Model file for the job. Use its own axes, mm. Face numbers are marked on the shaded views. A direction names the side the tool comes from. Round coordinates to 2 decimals unless told otherwise and drop trailing zeros. Loops run counter-clockwise (first coordinate to the right, second up) from the corner with the lowest first, then second, coordinate; pieces in that order, holes last. Notation, with made-up numbers: M 84,-19.75 L 97,-19.75 A13 ccw 97,4.25 Z; hole C 3,16 d5. An arc over 180 degrees is marked long. Use a Markdown table: item, result. Add a question column.
Q1. Mould opens along Y. For the marked faces 1, 2 and 3 say: +Y half, -Y half, draft (parallel to the pull), parting line (faces both ways), or undercut.
Q2. Cut at A-A (z = 17). Give the cut face in (x, y).
Q3. Cut at B-B (y = 10). Give the cut face in (x, z).
Q4. Cut at C-C (x = 131). Give the cut face in (y, z), plus the area to 3 significant figures.
Q5. Probe line 1 (Y direction, x = 25, z = 54); line 2 (X direction, y = 14.5, z = 6); line 3 (Z direction, x = 43, y = 40). List the from-to ranges inside material, lowest first. Write a range as from..to.
Q6. Tool access for the marked faces 4, 5, 6, 7 and 8: list every direction of +Z, -Z, +X, -X, +Y, -Y with a clear straight run to the whole face (end or side of a thin tool).
Q7. Pin check, flat tips, straight feed: pin 1 (6 mm diameter, centred on y = 31.5, z = 79, fed in from +X); pin 2 (20.5 mm diameter, centred on y = 28.5, z = 11.5, fed in from +X); pin 3 (9.5 mm diameter, centred on x = 78.5, y = 25.5, fed in from -Z); pin 4 (12 mm diameter, centred on x = 118.5, y = 7, fed in from -Z). Stop position of each tip, or through.
Q8. Cut at D-D (y = 47.5). Give the cut face in (x, z).
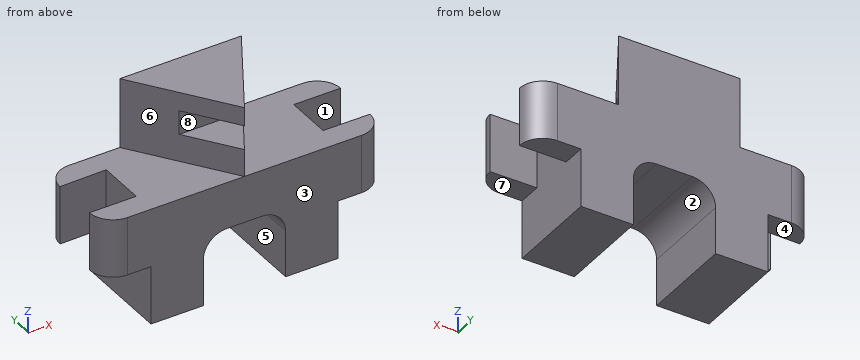
from build123d import *

# Parameters (mm, degrees)
F2_DEPTH = 50.8
F3_DEPTH = 63.5
F5_START = 38.1
F5_DEPTH = 63.5
F6_W     = 26.5905056149
F6_H     = 13.1163969636
F7_DEPTH = 152.401


with BuildPart() as f2:
    # F0 (on Front) → F2 (new body)
    with BuildSketch(Plane.XZ):
        with BuildLine():
            Line((25.4, 31.75), (25.4, 0))
            Line((25.4, 0), (53.848, 0))
            Line((53.848, 0), (53.848, 25.4))
            ThreePointArc((53.848, 25.4), (57.5677438789, 34.3802561211), (66.548, 38.1))
            Line((66.548, 38.1), (85.852, 38.1))
            ThreePointArc((85.852, 38.1), (94.8322561211, 34.3802561211), (98.552, 25.4))
            Line((98.552, 25.4), (98.552, 0))
            Line((98.552, 0), (127, 0))
            Line((127, 0), (127, 31.75))
            Line((127, 31.75), (152.4, 31.75))
            Line((152.4, 31.75), (152.4, 63.5))
            Line((152.4, 63.5), (127, 63.5))
            Line((127, 63.5), (88.9, 63.5))
            Line((88.9, 63.5), (63.5, 63.5))
            Line((63.5, 63.5), (38.1, 63.5))
            Line((38.1, 63.5), (25.4, 63.5))
            Line((25.4, 63.5), (0, 63.5))
            Line((0, 63.5), (0, 31.75))
            Line((0, 31.75), (25.4, 31.75))
        make_face()
    extrude(amount=-F2_DEPTH)

    # F1 (on Top) → F3 (cut)
    with BuildSketch(Plane.XY):
        with BuildLine():
            Line((0, 50.8), (0, 38.1))
            ThreePointArc((0, 38.1), (3.7197438789, 47.0802561211), (12.7, 50.8))
            Line((12.7, 50.8), (0, 50.8))
        make_face()
        with BuildLine():
            ThreePointArc((12.7, 0), (3.7197438789, 3.7197438789), (0, 12.7))
            Line((0, 12.7), (0, 0))
            Line((0, 0), (12.7, 0))
        make_face()
        Polygon((0, 38.1), (0, 12.7), (25.4, 12.7), (25.4, 38.5738648474), align=None)
        Polygon((127, 12.8180403262), (152.4, 12.7), (152.4, 38.1), (127, 38.1), align=None)
        with BuildLine():
            Line((152.4, 0), (152.4, 12.7))
            ThreePointArc((152.4, 12.7), (148.6802561211, 3.7197438789), (139.7, 0))
            Line((139.7, 0), (152.4, 0))
        make_face()
        with BuildLine():
            ThreePointArc((139.7, 50.8), (148.6802561211, 47.0802561211), (152.4, 38.1))
            Line((152.4, 38.1), (152.4, 50.8))
            Line((152.4, 50.8), (139.7, 50.8))
        make_face()
    extrude(amount=F3_DEPTH, mode=Mode.SUBTRACT)

    # F4 (on Top) → F5 (join)
    with BuildSketch(Plane.XY.offset(F5_START)):
        Polygon((40.4607152585, 50.8), (76.2, 0), (106.5007152585, 50.8), align=None)
    extrude(amount=F5_DEPTH)

    # F6 (on Right) → F7 (cut, through all)
    with BuildSketch(Plane.YZ):
        with Locations((13.2952528074, 84.9594064057)):
            Rectangle(F6_W, F6_H)
    extrude(amount=F7_DEPTH, mode=Mode.SUBTRACT)


solid = f2.part
Checked values:
| question | item | result |
|---|---|---|
| 1 | face 1 | undercut |
| 1 | face 2 | draft |
| 1 | face 3 | -Y half |
| 2 | outline | M 25.4,0 L 53.85,0 L 53.85,50.8 L 25.4,50.8 Z; M 98.55,0 L 127,0 L 127,50.8 L 98.55,50.8 Z |
| 3 | outline | M 0.29,31.75 L 25.4,31.75 L 25.4,0 L 53.85,0 L 53.85,25.4 A12.7 cw 66.55,38.1 L 85.85,38.1 A12.7 cw 98.55,25.4 L 98.55,0 L 127,0 L 127,31.75 L 152.11,31.75 L 152.11,63.5 L 82.16,63.5 L 82.16,78.4 L 69.16,78.4 L 69.16,63.5 L 0.29,63.5 Z; M 69.16,91.52 L 82.16,91.52 L 82.16,101.6 L 69.16,101.6 Z |
| 4 | outline | M 0,31.75 L 12.8,31.75 L 12.8,63.5 L 0,63.5 Z; M 38.1,31.75 L 50.8,31.75 L 50.8,63.5 L 38.1,63.5 Z |
| 4 | area | 810 mm^2 |
| 5 | line 1 | y = 0..12.7, 38.57..50.8 |
| 5 | line 2 | x = 25.4..53.85, 98.55..127 |
| 5 | line 3 | z = 0..63.5 |
| 6 | face 4 | -Z, -X, +Y, -Y |
| 6 | face 5 | -Z, +Y, -Y |
| 6 | face 6 | +Z, -X, -Y |
| 6 | face 7 | -Z, +X, +Y, -Y |
| 6 | face 8 | +X, -X, -Y |
| 7 | pin 1 | stops at x = 96.78 |
| 7 | pin 2 | stops at x = 127 |
| 7 | pin 3 | stops at z = 38.1 |
| 7 | pin 4 | stops at z = 0 |
| 8 | outline | M 4.16,31.75 L 25.4,31.75 L 25.4,0 L 53.85,0 L 53.85,25.4 A12.7 cw 66.55,38.1 L 85.85,38.1 A12.7 cw 98.55,25.4 L 98.55,0 L 127,0 L 127,31.75 L 148.24,31.75 L 148.24,63.5 L 104.53,63.5 L 104.53,101.6 L 42.78,101.6 L 42.78,63.5 L 4.16,63.5 Z |
